from build123d import *

# Parameters (mm, degrees)
F0_W     = 457.2
F0_H     = 254
F0_R     = 9.525
F0_R_2   = 15.875
F0_R_3   = 11.1125
F1_DEPTH = 19.05


with BuildPart() as f1:
    # F0 (on Top) → F1 (new body)
    with BuildSketch(Plane.XY):
        Rectangle(F0_W, F0_H)
        with Locations((-34.5948, -59.5376)):
            Circle(F0_R, mode=Mode.SUBTRACT)
        with Locations((34.5948, -59.5376)):
            Circle(F0_R, mode=Mode.SUBTRACT)
        with Locations((-177.8, 0)):
            Circle(F0_R_2, mode=Mode.SUBTRACT)
        with Locations((-34.5948, 59.5376)):
            Circle(F0_R, mode=Mode.SUBTRACT)
        Circle(F0_R_3, mode=Mode.SUBTRACT)
        with Locations((34.5948, 59.5376)):
            Circle(F0_R, mode=Mode.SUBTRACT)
        with Locations((177.8, 0)):
            Circle(F0_R_2, mode=Mode.SUBTRACT)
    extrude(amount=F1_DEPTH)


solid = f1.part
Build history of the part. All positions in model axes, mm. Round coordinates to 2 decimals unless told otherwise and drop trailing zeros. Order: outer loops, then holes, each group sorted by start corner. A loop starts at its lowest first (then second) coordinate and runs counter-clockwise, first axis right, second up. Notation, with made-up numbers: M 53,-32.5 L 85,-32.5 A9 cw 85,-18.5 Z; hole C 16.5,16.5 d7. An arc over 180 degrees is marked long. Use CSV: the item, a comma, the result in double quotes. Start each with the question number.
(1) Flat gauge pins, fed straight in: P1, Ø22, axis at x = 34.59, y = -59.54, coming from the +Z side; P2, Ø17, axis at x = -34.59, y = 59.54, coming from the +Z side. Where does each tip first touch, or does it go through?
(2) Cut at C-C on x = 177.8. List the corners of the cut face in (y, z) (3 decimals).
(3) Drill centre lines: probe 1 along Y at (x, z) = (177.8, 14) (3 decimals); probe 2 along Y at (x, z) = (-37.5, 17.5); probe 3 along X at (y, z) = (-67, 7.5). Where is each one in solid material? Low to high.
(4) Mould opens along X. For faces 1 (the face through (-228.6, -2, 9)), 2 (the face through (10.6, 3.34, 9.39)), 3 (the face through (-3, 127, 9)) say: +X half, -X half, draft (parallel to the pull), parting line (faces both ways), or undercut.
(5) Cut at A-A on x = 0. List the corners of the cut face in (y, z), then the cut area to 3 significant figures.
(6) Cut at B-B on y = 0. State how many separate pieces and enclosed holes the cut face has, then the cut area to 3 significant figures.
Findings:
1,P1,"stops at z = 19.05"
1,P2,"passes through"
2,outline,"M -127,0 L -15.875,0 L -15.875,19.05 L -127,19.05 Z; M 15.875,0 L 127,0 L 127,19.05 L 15.875,19.05 Z"
3,probe 1,"y = -127 to -15.875, 15.875 to 127"
3,probe 2,"y = -127 to -68.61, -50.47 to 50.47, 68.61 to 127"
3,probe 3,"x = -228.6 to -40.51, -28.68 to 28.68, 40.51 to 228.6"
4,face 1,"-X half"
4,face 2,"undercut"
4,face 3,"draft"
5,outline,"M -127,0 L -11.11,0 L -11.11,19.05 L -127,19.05 Z; M 11.11,0 L 127,0 L 127,19.05 L 11.11,19.05 Z"
5,area,"4,420 mm^2"
6,separate pieces,"4"
6,enclosed holes,"0"
6,area,"7,080 mm^2"
